Autodesk Inventor part; units mm, degrees
ref_plane "Work Plane5" through (27, -19.0453, 1) normal (0, -1, 0) x (1, 0, 0)
ref_plane "Work Plane6" through (0, 56.5, 0) normal (0, 1, 0) x (-1, 0, 0)
ref_plane "YZ Plane" through (0, 0, 0) normal (1, 0, 0) x (0, 1, 0)
sketch "Sketch1" plane through (0, 0, 0) normal (0, 0, 1) x (1, 0, 0)
  line L0 (-14.081, 0) -> (14.081, 0) construction
  line L1 (0, -22) -> (0, 22) construction
  arc A0 (12.8558, 37.3209) -> (-12.8558, 37.3209) centre (0, 22) ccw
  line L2 (-65.2139, 3.8302) -> (-4.8209, 54.5062)
  arc A1 (4.8209, 54.5062) -> (-4.8209, 54.5062) centre (0, 48.7609) ccw
  line L3 (4.8209, 54.5062) -> (65.2139, 3.8302)
  arc A2 (63.607, -4.7347) -> (65.2139, 3.8302) centre (62, 0) ccw
  line L4 (63.607, -4.7347) -> (35.393, -14.3106)
  arc A3 (35.393, -14.3106) -> (32, -19.0453) centre (37, -19.0453) ccw
  line L5 (32, -19.0453) -> (32, -21.0453) construction
  line L6 (27, -21.0453) -> (27, -19.0453) construction
  arc A4 (33.7861, -9.5759) -> (27, -19.0453) centre (37, -19.0453) ccw
  line L7 (33.7861, -9.5759) -> (53.6299, -2.8408)
  arc A5 (53.6299, -2.8408) -> (54.5941, 2.2981) centre (52.6657, 0) ccw
  line L8 (54.5941, 2.2981) -> (12.8558, 37.3209)
  line L9 (-12.8558, 37.3209) -> (-54.5941, 2.2981)
  arc A6 (-54.5941, 2.2981) -> (-53.6299, -2.8408) centre (-52.6657, 0) ccw
  line L10 (-53.6299, -2.8408) -> (-33.7861, -9.5759)
  arc A7 (-27, -19.0453) -> (-33.7861, -9.5759) centre (-37, -19.0453) ccw
  line L11 (-27, -19.0453) -> (-27, -21.0453) construction
  line L12 (-32, -21.0453) -> (-32, -19.0453) construction
  arc A8 (-32, -19.0453) -> (-35.393, -14.3106) centre (-37, -19.0453) ccw
  line L13 (-35.393, -14.3106) -> (-63.607, -4.7347)
  arc A9 (-65.2139, 3.8302) -> (-63.607, -4.7347) centre (-62, 0) ccw
  line L14 (-32, -19.0453) -> (-27, -19.0453)
  line L15 (32, -19.0453) -> (27, -19.0453)
  point P0 (0, 0)
  point P1 (0, 0)
  point P2 (-29.5, -21.0453)
  point P3 (29.5, -21.0453)
  dimension "d0" = 40
  dimension "d1" = 22
  dimension "d2" = 8
  dimension "d3" = 3
  dimension "d4" = 3
  dimension "d5" = 5
  dimension "d6" = 5
  dimension "d7" = 5
  dimension "d8" = 5
  dimension "d9" = 7.5
  dimension "d10" = 8
  dimension "d11" = 124
  dimension "d12" = 62
  dimension "d13" = 10
  dimension "d14" = 5
  dimension "d15" = 10
  dimension "d16" = 5
  dimension "d17" = 5
  dimension "d18" = 48.7609
  dimension "d20" = 29.5
  dimension "d21" = 59
extrude "Extrusion1" add sketch "Sketch1" along normal mid plane 2
ref_plane "Work Plane5" through (27, -19.0453, 1) normal (0, -1, 0) x (1, 0, 0)
sketch "Sketch5" plane through (27, -19.0453, 1) normal (0, -1, 0) x (1, 0, 0)
  line L0 (-54, -2) -> (-59, -2)
  line L1 (-54, -2) -> (-54, 0)
  line L2 (-59, 0) -> (-54, 0)
  line L3 (-59, -2) -> (-59, 0)
  line L4 (-54, -2) -> (-59, -2)
  line L5 (5, -2) -> (5, 0)
  line L6 (0, 0) -> (5, 0)
  line L7 (0, 0) -> (0, -2)
  line L8 (5, -2) -> (0, -2)
  line L9 (0, 0) -> (5, 0)
  line L10 (5, 0) -> (5, 4)
  arc A0 (5, 4) -> (0, 4) centre (2.5, 4) ccw
  line L11 (0, 4) -> (0, 0)
  line L12 (38.2139, 0) -> (-22.1791, 0)
  line L13 (-54, 0) -> (-54, 4)
  arc A1 (-54, 4) -> (-59, 4) centre (-56.5, 4) ccw
  line L14 (-59, 4) -> (-59, 0)
  point P0 (-27, -1)
  dimension "d29" = 2.5
  dimension "d30" = 2.5
  dimension "d31" = 4
  dimension "d32" = 4
extrude "Extrusion2" add sketch "Sketch5" along normal blind 2
fillet "Fillet3" radius 1 2 edges at (-29.5, -19.0453, 1) (29.5, -19.0453, 1)
fillet "Fillet4" radius 3 2 edges at (-29.5, -21.0453, -1) (29.5, -21.0453, -1)
sketch "Sketch7" plane through (27, -19.0453, 1) normal (0, 1, 0) x (1, 0, 0)
  arc A0 (-59, -4) -> (-54, -4) centre (-56.5, -4) ccw
  arc A1 (0, -4) -> (5, -4) centre (2.5, -4) ccw
  point P0 (-27, 1)
hole "Hole2" at (-29.5, -19.0453, 5) at (29.5, -19.0453, 5) direction (0, -1, 0) diameter 3 depth 2
sketch "Sketch8" plane through (0, 0, 1) normal (0, 0, 1) x (1, 0, 0)
  arc A0 (-65.2139, 3.8302) -> (-63.607, -4.7347) centre (-62, 0) ccw
  arc A1 (63.607, -4.7347) -> (65.2139, 3.8302) centre (62, 0) ccw
  point P0 (0, 0)
hole "Hole3" at (-62, 0, 1) at (62, 0, 1) direction (0, 0, -1) diameter 4 depth 2
sketch "Sketch9" plane through (0, 0, 1) normal (0, 0, 1) x (1, 0, 0)
  arc A0 (4.8209, 54.5062) -> (-4.8209, 54.5062) centre (0, 48.7609) ccw
  point P0 (0, 0)
hole "Hole4" at (0, 48.7609, 1) direction (0, 0, -1) diameter 8 depth 2
ref_plane "Work Plane6" through (0, 56.5, 0) normal (0, 1, 0) x (-1, 0, 0)
sketch "Sketch10" plane through (0, 56.5, 0) normal (0, 1, 0) x (-1, 0, 0)
  point P0 (0, 0)
  point P1 (0, 0)
hole "Hole5" at (0, 56.5, 0) direction (0, -1, 0) diameter 1 depth 4
equation "\"d4\" = d3"
equation "\"d6\" = d5"
equation "\"d10\" = d2"
equation "\"d15\" = d13"
equation "\"d16\" = d14"
equation "\"d32\" = d31"
properties part number "01"
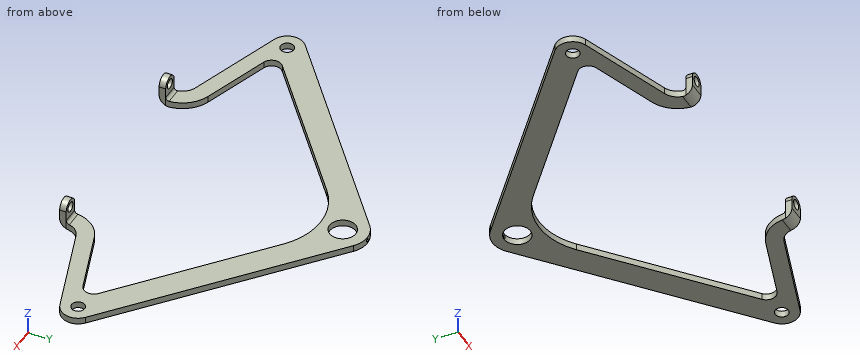
Here's how the part is built. I have some questions about the finished solid (model axes, mm). Give positions to 0.01 mm unless a question says otherwise; leave off trailing zeros. Write each loop counter-clockwise with the first axis right and the second up, starting at its lowest first coordinate (ties: lowest second). Pieces come first, ordered by that corner, then holes. Notation, with made-up numbers: M -9.75,-28.75 L 15.25,-28.75 A17 cw 15.25,-1.75 Z; hole C -11,-26 d10. An arc over 180 degrees is marked long. Put each result on its own line as item: value. Start each with the question number.
Item 1: If we section it at C-C, the plane x = 29.5: Write out the boundary of the cut face in (y, z).
Item 2: If we section it at A-A, the plane y = 0: Write out the boundary of the cut face in (x, z).
Item 3: If we section it at B-B, the plane x = 62: Write out the boundary of the cut face in (y, z), then the cut area to 3 significant figures.
Item 4: I need wall thicknesses on L1, parallel to X at y = 0, z = 0.5; L2, parallel to Y at x = 62, z = -0.55; L3, parallel to X at y = -18, z = 0.5. Which ranges of each line are inside material? Lowest first, please. Write a range as from..to.
Item 5: If we section it at D-D, the plane y = 21.5: Write out the boundary of the cut face in (x, z), then the cut area to 3 significant figures.
Item 6: Will these pins go through, and if not, where does the flat tip stop? pin 1 (3.5 mm diameter, centred on x = 29.5, z = 5, fed in from +Y); pin 2 (0.6 mm diameter, centred on y = -20.5, z = 1, fed in from -X); pin 3 (1.6 mm diameter, centred on y = -20, z = 0.5, fed in from +X).
Values:
1. outline: M -21.05,2 A3 ccw -18.05,-1 L -12.43,-1 L -12.43,1 L -18.05,1 A1 cw -19.05,2 L -19.05,3.5 L -21.05,3.5 Z; M -21.05,6.5 L -19.05,6.5 L -19.05,7.5 L -21.05,7.5 Z; M 23.35,-1 L 33.8,-1 L 33.8,1 L 23.35,1 Z
2. outline: M -67,-1 L -64,-1 L -64,1 L -67,1 Z; M -60,-1 L -55.67,-1 L -55.67,1 L -60,1 Z; M 55.67,-1 L 60,-1 L 60,1 L 55.67,1 Z; M 64,-1 L 67,-1 L 67,1 L 64,1 Z
3. outline: M -5.28,-1 L -2,-1 L -2,1 L -5.28,1 Z; M 2,-1 L 6.53,-1 L 6.53,1 L 2,1 Z
3. area: 15.6 mm²
4. L1: -67..-64, -60..-55.67, 55.67..60, 64..67
4. L2: -5.28..-2, 2..6.53
4. L3: -32.11..-27.05, 27.05..32.11
5. outline: M -44.16,-1 L -31.71,-1 L -31.71,1 L -44.16,1 Z; M 31.71,-1 L 44.16,-1 L 44.16,1 L 31.71,1 Z
5. area: 49.8 mm²
6. pin 1: y = -19.05
6. pin 2: x = -32
6. pin 3: x = 32
